Part model, mm, in its own coordinate system. A direction names the side the tool comes from. Give positions to 0.01 mm unless a question says otherwise; leave off trailing zeros. Answer as a JSON object with one key per item and string values.
from build123d import *

# Parameters (mm, degrees)
F1_DEPTH = 6.35
F2_R     = 2.54
F3_R     = 1.016
F4_R     = 0.762
F5_SIZE  = 0.508
F6_W     = 0.762
F6_H     = 31.75
F7_DEPTH = 0.762
F8_W     = 0.762
F8_H     = 0.7506295204
F8_H_2   = 0.762
F9_DEPTH = 25.4
F10_R    = 0.12699


# Not quite as in the source:
# - a fillet or chamfer is up to 0.001 mm smaller than in the source, because OpenCascade refuses the exact size


with BuildPart() as f1:
    # F0 (on Top) → F1 (new body)
    with BuildSketch(Plane.XY):
        Polygon((0, -14.2875), (0, 14.2875), (-4.064, 14.2875), (-5.3975, 2.8575), (-20.6375, 3.556), (-20.6375, -3.556), (-5.3975, -2.8575), (-4.064, -14.2875), align=None)
    extrude(amount=F1_DEPTH)

    # F2
    f2_edges = [f1.edges().sort_by_distance(p)[0] for p in [
        (-5.3975, -2.8575, 3.175),
        (-5.3975, 2.8575, 3.175),
    ]]
    fillet(f2_edges, radius=F2_R)

    # F3
    f3_edges = [f1.edges().sort_by_distance(p)[0] for p in [
        (0, 14.2875, 3.175),
        (-4.064, 14.2875, 3.175),
        (0, -14.2875, 3.175),
        (-4.064, -14.2875, 3.175),
        (-20.6375, 3.556, 3.175),
        (-20.6375, -3.556, 3.175),
    ]]
    fillet(f3_edges, radius=F3_R)

    # F4
    f4_edges = [f1.edges().sort_by_distance(p)[0] for p in [
        (-4.645984, 9.299062, 6.35),
        (-3.835156, 14.030405, 6.35),
        (-6.001163, 3.567789, 6.35),
        (-2.087821, 14.2875, 6.35),
        (-13.668668, 3.236595, 6.35),
        (-0.29758, 13.98992, 6.35),
        (-20.323281, 3.22705, 6.35),
        (0, 0, 6.35),
        (-20.6375, 0, 6.35),
        (-0.29758, -13.98992, 6.35),
        (-20.323281, -3.22705, 6.35),
        (-2.087821, -14.2875, 6.35),
        (-13.668668, -3.236595, 6.35),
        (-3.835156, -14.030405, 6.35),
        (-6.001163, -3.567789, 6.35),
        (-4.645984, -9.299062, 6.35),
    ]]
    fillet(f4_edges, radius=F4_R)

    # F5
    f5_edges = [f1.edges().sort_by_distance(p)[0] for p in [
        (-4.645984, 9.299062, 0),
        (-3.835156, 14.030405, 0),
        (-6.001163, 3.567789, 0),
        (-2.087821, 14.2875, 0),
        (-13.668668, 3.236595, 0),
        (-0.29758, 13.98992, 0),
        (-20.323281, 3.22705, 0),
        (0, 0, 0),
        (-20.6375, 0, 0),
        (-0.29758, -13.98992, 0),
        (-20.323281, -3.22705, 0),
        (-2.087821, -14.2875, 0),
        (-13.668668, -3.236595, 0),
        (-3.835156, -14.030405, 0),
        (-6.001163, -3.567789, 0),
        (-4.645984, -9.299062, 0),
    ]]
    chamfer(f5_edges, length=F5_SIZE)

    # F6 (on face) → F7 (cut)
    with BuildSketch(Plane.XY.offset(6.35)):
        with Locations((-1.524, -0.5830885321)):
            Rectangle(F6_W, F6_H)
    extrude(amount=-F7_DEPTH, mode=Mode.SUBTRACT)

    # F8 (on face) → F9 (cut)
    with BuildSketch(Plane.XY.offset(5.588)):
        with Locations((-1.524, 13.9121852398)):
            Rectangle(F8_W, F8_H)
        with Locations((-1.524, -13.9065)):
            Rectangle(F8_W, F8_H_2)
    extrude(amount=-F9_DEPTH, mode=Mode.SUBTRACT)

    # F10 (radius 0.127 in the source; OpenCascade refuses exactly that, so slightly less here)
    f10_edges = [f1.edges().sort_by_distance(p)[0] for p in [
        (-1.143, 0, 6.35),
        (-1.905, 0, 6.35),
    ]]
    fillet(f10_edges, radius=F10_R)


solid = f1.part
1. Which spindle directions (+Z, -Z, +X, -X, +Y, -Y) get a long thin tool onto all of the face, cutting with end or side? Do faces 1 (the flat face through (-4.38, 9.33, 0.25)), 2 (the cylindrical face through (-6.02, -3.55, 3.08)). Say none if no direction does.
Worked answers:
{"face 1": "-Z, -X, +Y", "face 2": "+Z, -Z, -Y"}
2. Two-plate mould, pull along X, no slides. Class faces 3 (the flat face through (-3, 14.288, 3)), 4 (the flat face through (-1.143, 0, 6)), 5 (the cylindrical face through (-3.827, -14.037, 3.084)), 6 (the flat face through (-1.905, 0, 6)): +X half, -X half, draft (parallel to the pull), parting line (faces both ways), or undercut.
Worked answers:
{"face 3": "draft", "face 4": "undercut", "face 5": "-X half", "face 6": "undercut"}
3. Probe line 1 along Y through (x, z) = (-3.25, 3.5); line 2 along Z through (x, y) = (-1.75, -4.5); line 3 along Y through (x, z) = (-7.5, 5). List the from-to ranges inside material, lowest first.
Worked answers:
{"line 1": "y = -14.28 to 14.28", "line 2": "z = 0 to 5.59", "line 3": "y = -2.97 to 2.97"}
4. Pin check, flat tips, straight feed: P1, Ø2, axis at x = -12, z = 3.5, coming from the +Y side; P2, Ø1.5, axis at x = -14.5, z = 5.5, coming from the -Y side; P3, Ø1.9, axis at y = 4, z = 2.5, coming from the -X side. Stop position of each tip, or through.
Worked answers:
{"P1": "stops at y = 3.21", "P2": "stops at y = -3.31", "P3": "stops at x = -20.47"}
